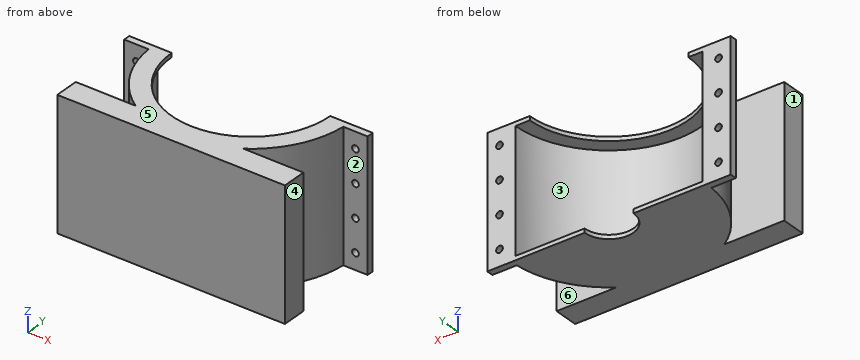
```python
from build123d import *

# Parameters (mm, degrees)
BOSS_EXTRUDE1_DEPTH = 8
CUT_EXTRUDE1_DEPTH  = 3.75
CUT_EXTRUDE2_DEPTH  = 3.75
CUT_EXTRUDE3_DEPTH  = 3.75
SKETCH7_R           = 0.205
CUT_EXTRUDE5_DEPTH  = 2


with BuildPart() as part:
    # Sketch1 → Boss-Extrude1 (new body)
    with BuildSketch(Plane.XY):
        with BuildLine():
            Line((-7, 0), (7, 0))
            Line((7, 0), (7, 1.5))
            Line((7, 1.5), (3.31662479, 1.5))
            ThreePointArc((3.31662479, 1.5), (5.186676874, 3.483647401), (5.985975276, 6.09))
            Line((5.985975276, 6.09), (7.485975276, 6.09))
            Line((7.485975276, 6.09), (7.485975276, 6.5))
            Line((7.485975276, 6.5), (4.875, 6.5))
            Line((4.875, 6.5), (-4.875, 6.5))
            Line((-4.875, 6.5), (-7.485975276, 6.5))
            Line((-7.485975276, 6.5), (-7.485975276, 6.09))
            Line((-7.485975276, 6.09), (-5.985975276, 6.09))
            ThreePointArc((-5.985975276, 6.09), (-5.186676874, 3.483647401), (-3.31662479, 1.5))
            Line((-3.31662479, 1.5), (-7, 1.5))
            Line((-7, 1.5), (-7, 0))
        make_face()
    extrude(amount=BOSS_EXTRUDE1_DEPTH)

    # Sketch3 → Cut-Extrude1 (cut, symmetric)
    with BuildSketch(Plane.XY.offset(4)):
        with BuildLine():
            Line((5.75, 6.5), (-5.75, 6.5))
            ThreePointArc((-5.75, 6.5), (0, 0.75), (5.75, 6.5))
        make_face()
    extrude(amount=CUT_EXTRUDE1_DEPTH, both=True, mode=Mode.SUBTRACT)

    # Sketch4 → Cut-Extrude2 (cut, symmetric)
    with BuildSketch(Plane.XY.offset(8)):
        with BuildLine():
            Line((-4.875, 6.5), (4.875, 6.5))
            ThreePointArc((4.875, 6.5), (0, 1.625), (-4.875, 6.5))
        make_face()
    extrude(amount=CUT_EXTRUDE2_DEPTH, both=True, mode=Mode.SUBTRACT)

    # Sketch6 → Cut-Extrude3 (cut, symmetric)
    with BuildSketch(Plane.XY.offset(0.25)):
        with BuildLine():
            Line((-1.5, 6.5), (1.5, 6.5))
            ThreePointArc((1.5, 6.5), (0, 5), (-1.5, 6.5))
        make_face()
    extrude(amount=CUT_EXTRUDE3_DEPTH, both=True, mode=Mode.SUBTRACT)

    # Sketch7 → Cut-Extrude5 (cut)
    with BuildSketch(Plane(origin=(0, 6.5, 0), x_dir=(1, 0, 0), z_dir=(0, 1, 0))):
        with Locations(Location((6.735975276, -7, 0), (0, 0, 270))):
            Circle(SKETCH7_R)
        with Locations(Location((6.735975276, -5, 0), (0, 0, 270))):
            Circle(SKETCH7_R)
        with Locations(Location((6.735975276, -3, 0), (0, 0, 270))):
            Circle(SKETCH7_R)
        with Locations(Location((6.735975276, -1, 0), (0, 0, 270))):
            Circle(SKETCH7_R)
    cut_extrude5 = extrude(amount=-CUT_EXTRUDE5_DEPTH, mode=Mode.SUBTRACT)

    # Mirror1: Cut-Extrude5 across plane
    add(cut_extrude5.mirror(Plane(origin=(0, 0, 0), x_dir=(0, 0, 1), z_dir=(1, 0, 0))), mode=Mode.SUBTRACT)


solid = part.part
```
Design review of the part built by this model. Coordinates are the model's own, in mm. Face numbers are marked on the shaded views. A direction names the side the tool comes from. Coordinates: 2 decimals unless noted, no trailing zeros. Order: outer loops, then holes, each group sorted by start corner. A loop starts at its lowest first (then second) coordinate and runs counter-clockwise, first axis right, second up. Notation, with made-up numbers: (-6.75, 47) - (32.25, 47) arc R6 ccw to (32.25, 54) - close; hole circle Ø1 at (11.5, -13). An arc over 180 degrees is marked (long way). Answer in a Markdown table with one row per item.
(1) Consider section A-A on z = 5. State the section outline as (x, y) points.
Checked values:
| item | result |
|---|---|
| outline | (-7.49, 6.09) - (-6.94, 6.09) - (-6.94, 6.5) - (-7.49, 6.5) - close; (-7, 0) - (7, 0) - (7, 1.5) - (3.32, 1.5) arc R6 ccw to (5.99, 6.09) - (6.53, 6.09) - (6.53, 6.5) - (5.75, 6.5) arc R5.75 cw to (-5.75, 6.5) - (-6.53, 6.5) - (-6.53, 6.09) - (-5.99, 6.09) arc R6 ccw to (-3.32, 1.5) - (-7, 1.5) - close; (6.94, 6.09) - (7.49, 6.09) - (7.49, 6.5) - (6.94, 6.5) - close |
(2) Consider section D-D on z = 2.5. State the section outline as (x, y) points, plus the area to 3 significant figures.
Checked values:
| item | result |
|---|---|
| outline | (-7.49, 6.09) - (-5.99, 6.09) arc R6 ccw to (-3.32, 1.5) - (-7, 1.5) - (-7, 0) - (7, 0) - (7, 1.5) - (3.32, 1.5) arc R6 ccw to (5.99, 6.09) - (7.49, 6.09) - (7.49, 6.5) - (5.75, 6.5) arc R5.75 cw to (-5.75, 6.5) - (-7.49, 6.5) - close |
| area | 22.3 mm^2 |
(3) The part is to be moulded in two halves that separate along X. For the marked faces 1, 2, 3 and 4, say which applies: released by +X, released by -X, zero draft, split by the parting line, or undercut.
Checked values:
| item | result |
|---|---|
| face 1 | released by -X |
| face 2 | zero draft |
| face 3 | undercut |
| face 4 | released by +X |
(4) For the marked faces 5 and 6, list the 3-axis set-ups (+Z, -Z, +X, -X, +Y, -Y) from which the entire face can be reached by the end or side of a thin tool; tool diameter is ignored.
Checked values:
| item | result |
|---|---|
| face 5 | +Z, +X, -X, +Y, -Y |
| face 6 | +Z, -Z, +X |
(5) Clearance check with flat-ended pins moving along their axes: pin 1 (1.2 mm diameter, centred on y = 0.5, z = 4.5, fed in from +X); pin 2 (1 mm diameter, centred on x = 3, z = 3, fed in from +Y); pin 3 (1 mm diameter, centred on y = 3, z = 4, fed in from -X). State where each tip first meets the part, or that it passes through.
Checked values:
| item | result |
|---|---|
| pin 1 | x = 7 |
| pin 2 | y = 1.94 |
| pin 3 | x = -5.2 |
(6) Consider section C-C on x = 3.75. State the section outline as (y, z) points, plus the area to 3 significant figures.
Checked values:
| item | result |
|---|---|
| outline | (0, 0) - (1.5, 0) - (1.5, 8) - (0, 8) - close; (1.82, 0) - (6.5, 0) - (6.5, 0.25) - (2.14, 0.25) - (2.14, 7.75) - (3.39, 7.75) - (3.39, 8) - (1.82, 8) - close |
| area | 16.0 mm^2 |
(7) Consider section B-B on x = 0. State the section outline as (y, z) points (3 decimals).
Checked values:
| item | result |
|---|---|
| outline | (0, 0) - (5, 0) - (5, 0.25) - (0.75, 0.25) - (0.75, 7.75) - (1.625, 7.75) - (1.625, 8) - (0, 8) - close |
(8) Wall thickness on line 1 along X through (y, z) = (6.4, 5); line 2 along Z through (x, y) = (3, 2.5); line 3 along Y through (x, z) = (6.5, 5.75): over which ranges is each line inside the solid? List them lowest first. Write a range as from..to.
Checked values:
| item | result |
|---|---|
| line 1 | -7.49..-6.94, -6.53..-5.75, 5.75..6.53, 6.94..7.49 |
| line 2 | 0..0.25, 7.75..8 |
| line 3 | 0..1.5, 6.09..6.5 |
